from build123d import *

# Parameters (mm, degrees)
F0_R          = 18
F0_W          = 150
F0_H          = 3
F2_DEPTH      = 110.5
F2_DEPTH_BACK = 4.9
F1_W          = 100
F1_H          = 94
F3_DEPTH      = 192.9
F0_R_2        = 15
F4_DEPTH      = 105
F4_DEPTH_BACK = 5


with BuildPart() as f2:
    # F0 (on Front) → F2 (new body, two sides)
    with BuildSketch(Plane.XZ) as f2_sk:
        Polygon((0, 80), (0, 0), (150, 0), (150, 80), (128.5714285714, 80), (128.5714285714, 103), (107.1428571429, 103), (107.1428571429, 80), (85.7142857143, 80), (85.7142857143, 103), (64.2857142857, 103), (64.2857142857, 80), (42.8571428571, 80), (42.8571428571, 103), (21.4285714286, 103), (21.4285714286, 80), align=None)
        with Locations((50, 47)):
            Circle(F0_R, mode=Mode.SUBTRACT)
        with Locations((75, -1.5)):
            Rectangle(F0_W, F0_H)
    extrude(amount=-F2_DEPTH)
    extrude(f2_sk.sketch, amount=F2_DEPTH_BACK)

    # F1 (on Right) → F3 (intersect)
    with BuildSketch(Plane.YZ):
        with BuildLine():
            Line((100, 97), (0, 97))
            ThreePointArc((0, 97), (-2.1213203436, 96.1213203436), (-3, 94))
            Line((-3, 94), (-3, 0))
            ThreePointArc((-3, 0), (-2.1213203436, -2.1213203436), (0, -3))
            Line((0, -3), (100, -3))
            ThreePointArc((100, -3), (102.1213203436, -2.1213203436), (103, 0))
            Line((103, 0), (103, 94))
            ThreePointArc((103, 94), (102.1213203436, 96.1213203436), (100, 97))
        make_face()
        with Locations((50, 47)):
            Rectangle(F1_W, F1_H, mode=Mode.SUBTRACT)
    extrude(amount=F3_DEPTH, mode=Mode.INTERSECT)

    # F0 (on Front) → F4 (join, two sides)
    with BuildSketch(Plane.XZ) as f4_sk:
        with Locations((50, 47)):
            Circle(F0_R)
        with Locations((50, 47)):
            Circle(F0_R_2, mode=Mode.SUBTRACT)
    extrude(amount=-F4_DEPTH)
    extrude(f4_sk.sketch, amount=F4_DEPTH_BACK)


solid = f2.part
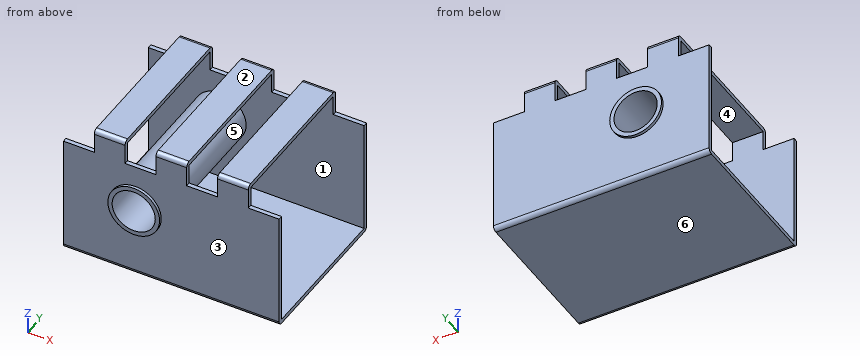
Can you work these out from the model? Positions are in its coordinate system, mm. Face numbers are marked on the shaded views. A direction names the side the tool comes from. Coordinates: 2 decimals unless noted, no trailing zeros. Loops run counter-clockwise (first coordinate to the right, second up) from the corner with the lowest first, then second, coordinate; pieces in that order, holes last. Notation, with made-up numbers: M -26.5,74 L -2.5,74 A14 ccw -2.5,101 Z; hole C -35,36 d10. An arc over 180 degrees is marked long. Return JSON: item names as keys, results as strings. Group by question number.
Item 1: Imagine slicing it at D-D (z = 85.5). Please give me the cut outline in (x, y).
Item 2: If I drill on L1, parallel to Z at x = 50, y = 83; L2, parallel to Y at x = 31.5, z = 7; L3, parallel to Z at x = 27.5, y = 56, over which ranges is the centre line in solid material (lowest first)? Write a range as from..to.
Item 3: Thinking about a two-plate mould opening in Z: for the marked faces 1, 2 and 3, which applies, released by +Z, released by -Z, zero draft, split by the parting line, or undercut?
Item 4: Imagine slicing it at B-B (y = 49). Please give me the cut outline in (x, z).
Item 5: Imagine slicing it at A-A (x = 50). Please give me the cut outline in (y, z), and give its area (3 significant figures).
Item 6: I'm going to push flat-ended pins straight in: pin 1 Ø1.5 at (x, y) = (142.5, -1) entering from +Z; pin 2 Ø18.5 at (y, z) = (73.5, 88) entering from +X; pin 3 Ø1 at (x, z) = (66, 60) entering from -Y; pin 4 Ø13.5 at (y, z) = (63, 85.5) entering from -X. Where does each tip first touch, or does it pass through?
Item 7: Imagine slicing it at C-C (z = 47). Please give me the cut outline in (x, y).
Item 8: On a 3-axis mill with a long thin cutter (end or side, diameter ignored), from which of +Z, -Z, +X, -X, +Y, -Y can I reach the whole of each face in a straight line? I mean the marked faces 4, 5 and 6. Say none if no direction works.
Verdict:
{
 "1": {"outline": "M 21.43,-3 L 42.86,-3 L 42.86,0 L 21.43,0 Z; M 21.43,100 L 42.86,100 L 42.86,103 L 21.43,103 Z; M 64.29,-3 L 85.71,-3 L 85.71,0 L 64.29,0 Z; M 64.29,100 L 85.71,100 L 85.71,103 L 64.29,103 Z; M 107.14,-3 L 128.57,-3 L 128.57,0 L 107.14,0 Z; M 107.14,100 L 128.57,100 L 128.57,103 L 107.14,103 Z"},
 "2": {"L1": "z = -3..0, 29..32, 62..65", "L2": "y = -3..0, 100..103", "L3": "z = -3..0, 94..97"},
 "3": {"face 1": "undercut", "face 2": "released by +Z", "face 3": "zero draft"},
 "4": {"outline": "M 0,-3 L 150,-3 L 150,0 L 0,0 Z; M 21.43,94 L 42.86,94 L 42.86,97 L 21.43,97 Z; C 50,47 d36; M 64.29,94 L 85.71,94 L 85.71,97 L 64.29,97 Z; M 107.14,94 L 128.57,94 L 128.57,97 L 107.14,97 Z; hole C 50,47 d30"},
 "5": {"outline": "M -5,29 L -3,29 L -3,0 A3 ccw 0,-3 L 100,-3 A3 ccw 103,0 L 103,29 L 105,29 L 105,32 L -5,32 Z; M -5,62 L 105,62 L 105,65 L 103,65 L 103,80 L 100,80 L 100,65 L 0,65 L 0,80 L -3,80 L -3,65 L -5,65 Z; hole M 0,0 L 100,0 L 100,29 L 0,29 Z", "area": "1,240 mm^2"},
 "6": {"pin 1": "stops at z = 80", "pin 2": "stops at x = 128.57", "pin 3": "stops at y = -3", "pin 4": "passes through"},
 "7": {"outline": "M 0,-3 L 32,-3 L 32,-5 L 35,-5 L 35,105 L 32,105 L 32,103 L 0,103 L 0,100 L 32,100 L 32,0 L 0,0 Z; M 65,-5 L 68,-5 L 68,-3 L 150,-3 L 150,0 L 68,0 L 68,100 L 150,100 L 150,103 L 68,103 L 68,105 L 65,105 Z"},
 "8": {"face 4": "+X, -X", "face 5": "none", "face 6": "-Z, +X, -X, +Y, -Y"}
}
